Geometry check sheet. Reference: drawing and pictorial views, mm from the part's lowest x, y, z. Coordinates: 2 decimals unless noted, no trailing zeros. Loops run counter-clockwise (first coordinate to the right, second up) from the corner with the lowest first, then second, coordinate; pieces in that order, holes last.
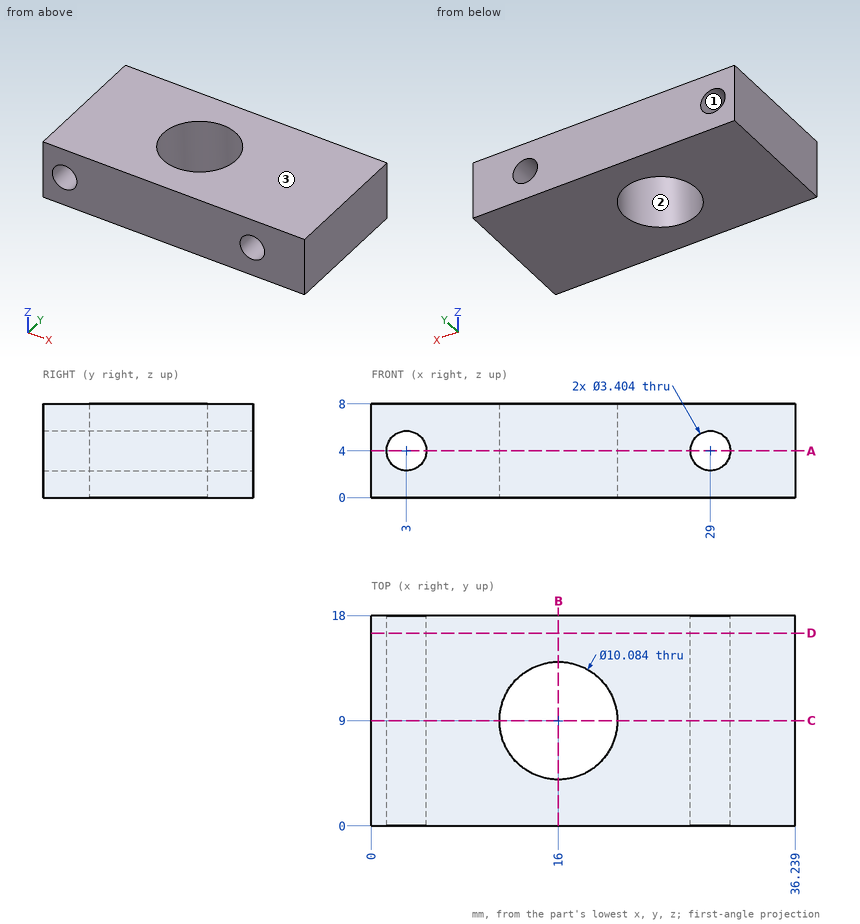
1) Section check B-B on x = 16. Record the cut outline in (y, z).
Data:
outline: (0, 0) - (3.96, 0) - (3.96, 8) - (0, 8) - close; (14.04, 0) - (18, 0) - (18, 8) - (14.04, 8) - close
2) Section check D-D on y = 16.5. Record the cut outline in (x, z).
Data:
outline: (0, 0) - (36.24, 0) - (36.24, 8) - (0, 8) - close; hole circle Ø3.4 at (3, 4); hole circle Ø3.4 at (29, 4)
3) Section check A-A on z = 4. Record the cut outline in (x, y).
Data:
outline: (0, 0) - (1.3, 0) - (1.3, 18) - (0, 18) - close; (4.7, 0) - (27.3, 0) - (27.3, 18) - (4.7, 18) - close; (30.7, 0) - (36.24, 0) - (36.24, 18) - (30.7, 18) - close; hole circle Ø10.08 at (16, 9)
4) Mould release check, pull along Z, two halves, no side actions. Record for the marked faces 1, 2 and 3: +Z half, -Z half, draft (parallel to the pull), parting line (faces both ways), or undercut.
Data:
face 1: undercut
face 2: draft
face 3: +Z half
5) Material ranges on probe 1 along X at (y, z) = (9.25, 4) (1 decimal); probe 2 along Y at (x, z) = (16, 5.75); probe 3 along X at (y, z) = (12.5, 4), recorded low to high.
Data:
probe 1: x = 0 to 1.3, 4.7 to 11, 21 to 27.3, 30.7 to 36.2
probe 2: y = 0 to 3.96, 14.04 to 18
probe 3: x = 0 to 1.3, 4.7 to 12.37, 19.63 to 27.3, 30.7 to 36.24
6) Section check C-C on y = 9. Record the cut outline in (x, z).
Data:
outline: (0, 0) - (10.96, 0) - (10.96, 8) - (0, 8) - close; (21.04, 0) - (36.24, 0) - (36.24, 8) - (21.04, 8) - close; hole circle Ø3.4 at (3, 4); hole circle Ø3.4 at (29, 4)
